Check sheet for the modelled part. Datum: model origin and axes. Units: mm. A direction names the side the tool comes from. Give positions to 0.01 mm unless a question says otherwise; leave off trailing zeros. Loops run counter-clockwise (first coordinate to the right, second up) from the corner with the lowest first, then second, coordinate; pieces in that order, holes last. Notation, with made-up numbers: M -21.75,82.25 L -17.75,82.25 A19 cw -17.75,92.25 Z; hole C 28,69 d7. An arc over 180 degrees is marked long. Write each question's results on one line, items separated by ' | '. Start each with the question number.
1. Material ranges on line 1 along Y through (x, z) = (0, -1.75); line 2 along Z through (x, y) = (-11, 10); line 3 along Z through (x, y) = (-3, -3.5), recorded low to high.
2. Sectioned sample at B-B on x = 0. Record the cut outline in (y, z).
3. Draft check along X on faces 1 (the flat face through (0, 1, 2.845)), 2 (the cylindrical face through (14.04, 7.93, 2.07)), 3 (the cylindrical face through (-4.817, -15.401, 2.068)), 4 (the cylindrical face through (-12.46, 0.34, 2.07)). Enter one of: pulls with the +X half, pulls with the -X half, needs draft (parallel to the pull), parting line crosses it, or undercut.
4. Sectioned sample at A-A on z = -4.5. Record the cut outline in (x, y), and give its area (3 significant figures).
5. Tool access check on faces 5 (the flat face through (8.527, -11.434, 2.046)), 6 (the flat face through (-5.13, 10.85, 2.05)), 7 (the cylindrical face through (-11.194, -5.566, 2.068)), 8 (the flat face through (-14.19, -0.24, 2.05)). Record the directions out of +Z, -Z, +X, -X, +Y, -Y that give a thin tool (end or side, any length) a straight path to the whole face; none if there is none.
6. Go/stop test with flat-tipped pins: pin 1 (2 mm diameter, centred on y = 0.5, z = -5.5, fed in from +X); pin 2 (5 mm diameter, centred on x = 7.5, z = 1.5, fed in from +Y); pin 3 (3 mm diameter, centred on x = 1.5, y = -1, fed in from -Z); pin 4 (3 mm diameter, centred on x = -2, z = -2.5, fed in from +Y). Record where each tip stops, or that it passes through.
7. Sectioned sample at C-C on y = 14. Record the cut outline in (x, z).
```python
from build123d import *

# Parameters (mm, degrees)
F1_DEPTH  = 2.54
F2_SCALE  = 1.12
F3_R      = 1.27
F4_R      = 4.0005
F4_R_2    = 2.1462999284
F5_DEPTH  = 7.0104
F6_R      = 2.2083863112
F7_DEPTH  = 7.0104
F8_DEPTH  = 1.27
F9_R      = 5.1360331122
F10_DEPTH = 1.27


with BuildPart() as f1:
    # F0 (on Top) → F1 (new body)
    with BuildSketch(Plane.XY):
        Polygon((2.6097216178, 14.5627437159), (-2.4016266689, 14.6046923473), (-2.4016266689, 10.7069099322), (-6.7973635159, 8.6464090273), (-9.7507489845, 11.1018400639), (-12.9371215583, 7.269280193), (-9.9187448393, 4.759815731), (-10.987800546, 0.1461525389), (-14.7898914292, -0.6685812259), (-13.7329729143, -5.6008676039), (-9.9187448393, -4.7835330123), (-6.9650523365, -8.5103949532), (-8.662414737, -11.9730141014), (-4.136644538, -14.1915290003), (-2.4166579341, -10.6827564792), (2.3025460541, -10.6827564792), (3.9659612812, -14.2644541338), (8.5153820935, -12.1516080526), (6.8819414162, -8.6344521752), (9.8897544667, -4.8440932296), (13.6239528656, -5.7776425965), (14.7675592452, -0.8934023208), (10.9942825511, -0.0382388607), (9.9505092949, 4.6697063372), (13.008704409, 7.0334360935), (9.9016642198, 10.9836040065), (6.8838195875, 8.5752755404), (2.5481330231, 10.6975259259), align=None)
    extrude(amount=F1_DEPTH)


with BuildPart() as f1_1:
    # F2: moved
    add(f1.part.scale(F2_SCALE))

    # F3
    f3_edges = [f1_1.edges().sort_by_distance(p)[0] for p in [
        (-16.564678, -0.748811, 1.4224),
        (-12.306337, 0.163691, 1.4224),
        (-14.489576, 8.141594, 1.4224),
        (-10.920839, 12.434061, 1.4224),
        (-7.613047, 9.683978, 1.4224),
        (-2.689822, 11.991739, 1.4224),
        (-2.689822, 16.357255, 1.4224),
        (2.922888, 16.310273, 1.4224),
        (2.853909, 11.981229, 1.4224),
        (7.709878, 9.604309, 1.4224),
        (11.089864, 12.301636, 1.4224),
        (14.569749, 7.877448, 1.4224),
        (11.14457, 5.230071, 1.4224),
        (12.313596, -0.042828, 1.4224),
        (16.539666, -1.000611, 1.4224),
        (15.258827, -6.47096, 1.4224),
        (11.076525, -5.425384, 1.4224),
        (7.707774, -9.670586, 1.4224),
        (9.537228, -13.609801, 1.4224),
        (4.441877, -15.976189, 1.4224),
        (2.578852, -11.964687, 1.4224),
        (-2.706657, -11.964687, 1.4224),
        (-4.633042, -15.894512, 1.4224),
        (-9.701905, -13.409776, 1.4224),
        (-7.800859, -9.531642, 1.4224),
        (-11.108994, -5.357557, 1.4224),
        (-15.38093, -6.272972, 1.4224),
        (-11.108994, 5.330994, 1.4224),
    ]]
    fillet(f3_edges, radius=F3_R)

    # F4 (on face) → F5 (join)
    with BuildSketch(Plane.XY):
        Circle(F4_R)
        Circle(F4_R_2, mode=Mode.SUBTRACT)
        Circle(F4_R_2)
    extrude(amount=-F5_DEPTH)

    # F6 (on face) → F7 (cut)
    with BuildSketch(Plane(origin=(0, 0, -7.0104), x_dir=(1, 0, 0), z_dir=(0, 0, -1))):
        Circle(F6_R)
    extrude(amount=-F7_DEPTH, mode=Mode.SUBTRACT)

    # F8 (cut): a face of the model
    f8_faces = [f1_1.faces().sort_by_distance(p)[0] for p in [
        (5.0824398182, 10.382465325, 0),
    ]]
    extrude(f8_faces, amount=-F8_DEPTH, mode=Mode.SUBTRACT)

    # F9 (on face) → F10 (join)
    with BuildSketch(Plane.XY):
        Circle(F9_R)
    extrude(amount=F10_DEPTH)


solid = f1_1.part
```
Output values:
1) line 1: -4 to -2.21, 2.21 to 4 | line 2: 1.27 to 2.84 | line 3: 0 to 2.84
2) outline: M -11.96,1.27 L -5.14,1.27 L -5.14,0 L -4,0 L -4,-7.01 L -2.21,-7.01 L -2.21,0 L 2.21,0 L 2.21,-7.01 L 4,-7.01 L 4,0 L 5.14,0 L 5.14,1.27 L 16.33,1.27 L 16.33,2.84 L -11.96,2.84 Z
3) face 1: needs draft | face 2: pulls with the +X half | face 3: undercut | face 4: pulls with the -X half
4) outline: C 0,0 d8; hole C 0,0 d4.42 | area: 35.0 mm2
5) face 5: +Z, -Z, +X | face 6: +Z, -Z, +Y | face 7: +Z, -Z, -Y | face 8: +Z, -Z, -X
6) pin 1: x = 4 | pin 2: y = 11.43 | pin 3: z = -7.01 | pin 4: y = 3.97
7) outline: M -2.69,1.27 L 2.89,1.27 L 2.89,2.84 L -2.69,2.84 Z
